Source: CAD feature listing. Evaluate the final solid. Frame: model axes, mm. A direction names the side the tool comes from. Give positions to 0.01 mm unless a question says otherwise; leave off trailing zeros. Loops run counter-clockwise (first coordinate to the right, second up) from the corner with the lowest first, then second, coordinate; pieces in that order, holes last. Notation, with made-up numbers: M 74.5,40 L 84.5,40 A13 ccw 84.5,65 Z; hole C -19.5,55 d5. An arc over 180 degrees is marked long. Answer in a Markdown table with one row per item.
Autodesk Fusion 360 part; units mm, degrees
sketch "Sketch1" plane through (0, 0, 0) normal (0, 0, 1) x (1, 0, 0)
  line L0 (0, 0) -> (0, 135)
  line L1 (0, 135) -> (8, 135)
  line L2 (8, 135) -> (8, 0)
  line L3 (8, 0) -> (0, 0)
  line L4 (8, 135) -> (8, 127) construction
  line L5 (8, 127) -> (16, 127)
  line L6 (16, 127) -> (16, 119)
  line L7 (16, 119) -> (8, 119)
  line L8 (8, 119) -> (8, 127)
  line L9 (4, 135) -> (4, 0) construction
  line L10 (12, 127) -> (8, 131)
  line L11 (12, 119) -> (8, 115)
  line L12 (12, 119) -> (12, 127) construction
  circle A0 centre (12, 123) radius 3.15
  line L13 (8, 131) -> (8, 115)
  dimension "d1" = 135
  dimension "d2" = 8
  dimension "d3" = 8
  dimension "d4" = 8
  dimension "d5" = 8
  dimension "d6" = 6.3
extrude "Extrude1" add sketch "Sketch1" along normal blind 20 contours L0 L1 L2 L3 L8 L13 makes body 1
extrude "Extrude2" add sketch "Sketch1" along normal blind 4 separate body contours L2 L7 L11 L13 | L2 L5 L10 L13 | L2 L5 L6 L7 L8 L13 makes body 2
pattern_linear "R-Pattern1" count 6 spacing 22 along (0, -1, 0) of bodies 2 makes body 3 at (15.1461, 100.843, 2.6667) makes body 4 at (15.1461, 78.843, 2.6667) makes body 5 at (8.8657, 56.6864, 2.6667) makes body 6 at (8.8657, 34.6864, 2.6667) makes body 7 at (15.1461, 12.843, 2.6667)
sketch "Sketch2" plane through (0, 0, 20) normal (0, 0, 1) x (-1, 0, 0)
  line L0 (-8, 0) -> (-8, -135)
  line L1 (-8, -135) -> (0, -135)
  line L2 (0, -135) -> (0, 0)
  line L3 (0, 0) -> (-8, 0)
  line L4 (-4, 0) -> (-4, -135)
ref_plane "WorkPlane1" through (4, 67.5, 10) normal (1, 0, 0) x (0, 1, 0)
mirror "Mirror1" about plane through (4, 67.5, 10) normal (1, 0, 0) of bodies 2 3 4 5 6 7 makes body 8 at (-7.1461, 122.843, 2.6667) makes body 9 at (-7.1461, 100.843, 2.6667) makes body 10 at (-7.1461, 78.843, 2.6667) makes body 11 at (-0.8657, 56.6864, 2.6667) makes body 12 at (-0.8657, 34.6864, 2.6667) makes body 13 at (-7.1461, 12.843, 2.6667)
combine "Combine1" operation add target body 1 tool bodies 8 9 10 11 12 13 6 7 5 4 3 2
Q1. Section query A-A (y = 123). Output: boundary loops of the cut face in (x, z).
Values follow:
| item | result |
|---|---|
| outline | M -8,0 L -7.15,0 L -7.15,4 L -8,4 Z; M -0.85,0 L 8.85,0 L 8.85,4 L 8,4 L 8,20 L 0,20 L 0,4 L -0.85,4 Z; M 15.15,0 L 16,0 L 16,4 L 15.15,4 Z |
Q2. Section query C-C (z = 8.5). Output: boundary loops of the cut face in (x, y), plus the area to 3 significant figures.
Values follow:
| item | result |
|---|---|
| outline | M 0,0 L 8,0 L 8,135 L 0,135 Z |
| area | 1,080 mm^2 |
Q3. Contact query for flat-ended pins moving along their axis: pin 1 Ø1.2 at (x, z) = (14.5, 2) entering from +Y; pin 2 Ø4.5 at (x, z) = (-5, 2) entering from -Y; pin 3 Ø4 at (x, y) = (12, 35) entering from +Z; pin 4 Ø1.5 at (y, z) = (18.5, 14) entering from +X. Output: stop coordinate, or through.
Values follow:
| item | result |
|---|---|
| pin 1 | y = 127 |
| pin 2 | y = 7.75 |
| pin 3 | through |
| pin 4 | x = 8 |
Q4. Mould query, pull axis Y, two halves, no side actions, for faces 1 (the flat face through (-6, 75, 2)), 2 (the flat face through (10, 129, 2)), 3 (the flat face through (16, 57, 2)). Classes: +Y half, -Y half, draft (parallel to the pull), parting line (faces both ways), or undercut.
Values follow:
| item | result |
|---|---|
| face 1 | undercut |
| face 2 | +Y half |
| face 3 | draft |
Q5. Reachability of faces 4 (the flat face through (-6, 105, 2)), 5 (the flat face through (14, 53, 2)), 6 (the flat face through (-1, 59, 4)) from +Z, -Z, +X, -X, +Y, -Y: full face, straight path, thin tool, end or side. Return the list, or none.
Values follow:
| item | result |
|---|---|
| face 4 | +Z, -Z, -X |
| face 5 | +Z, -Z, +X |
| face 6 | +Z, -X, +Y, -Y |
Q6. Section query D-D (y = 45.5). Output: boundary loops of the cut face in (x, z), plus the area to 3 significant figures.
Values follow:
| item | result |
|---|---|
| outline | M 0,0 L 8,0 L 8,20 L 0,20 Z |
| area | 160 mm^2 |
Q7. Section query B-B (y = 84.5). Output: boundary loops of the cut face in (x, z).
Values follow:
| item | result |
|---|---|
| outline | M -2.5,0 L 10.5,0 L 10.5,4 L 8,4 L 8,20 L 0,20 L 0,4 L -2.5,4 Z |
Q8. Ray query, probe 1 along X at (y, z) = (22, 14.75); probe 2 along X at (y, z) = (50, 2). Return the intervals inside material, ascending. Write a range as from..to.
Values follow:
| item | result |
|---|---|
| probe 1 | 0..8 |
| probe 2 | -1..9 |
